Verification items for the finished model (mm, model axes). Face numbers are marked on the shaded views. A direction names the side the tool comes from. Coordinates: 2 decimals unless noted, no trailing zeros. Order: outer loops, then holes, each group sorted by start corner. A loop starts at its lowest first (then second) coordinate and runs counter-clockwise, first axis right, second up. Notation, with made-up numbers: M -28.5,81 L -10.5,81 A27 cw -10.5,97 Z; hole C -22,33 d7. An arc over 180 degrees is marked long. Return JSON: item names as keys, results as strings. Group by question number.
1. Material ranges on line 1 along Y through (x, z) = (10, 2.5); line 2 along X through (y, z) = (-5.5, 10.5); line 3 along X through (y, z) = (-2.5, 3.5), recorded low to high.
2. Section check C-C, the plane y = -2.25. Record the cut outline in (x, z), plus the area to 3 significant figures.
3. Mould release check, pull along Y, two halves, no side actions. Record for the marked faces 5, 6 and 7: +Y half, -Y half, draft (parallel to the pull), parting line (faces both ways), or undercut.
4. Section check D-D, the plane x = -2. Record the cut outline in (y, z).
5. Section check B-B, the plane z = 8. Record the cut outline in (x, y).
6. Section check A-A, the plane x = -9.5. Record the cut outline in (y, z).
7. Set-up check for the marked faces 1, 2, 3 and 4: record each of +Z, -Z, +X, -X, +Y, -Y from which the full face is reachable in a straight line by a thin tool's end or side.
8. Gauge pin test, flat ends, axial feed: pin 1 (3 mm diameter, centred on x = -3, y = 2, fed in from +Z); pin 2 (7 mm diameter, centred on y = -3, z = 11, fed in from -X); pin 3 (1.2 mm diameter, centred on x = -10.5, y = 5, fed in from +Z). Record the tip position at first contact, or that the pin passes through.
```python
from build123d import *

# Parameters (mm, degrees)
SKETCH1_W               = 23.3
SKETCH1_H               = 15.5
BOSS_EXTRUDE1_DEPTH     = 3
SKETCH2_W               = 15.5
SKETCH2_H               = 15.5
BOSS_EXTRUDE2_DEPTH     = 10.5
CUT_EXTRUDE1_DEPTH      = 8
CUT_EXTRUDE2_DEPTH      = 10
CUT_EXTRUDE2_DEPTH_BACK = 3
SKETCH4_R               = 1.5
SKETCH5_W               = 35.704226427
SKETCH5_H               = 23.298790068
CUT_EXTRUDE3_DEPTH      = 1.6


with BuildPart() as part:
    # Sketch1 → Boss-Extrude1 (new body)
    with BuildSketch(Plane.XY):
        Rectangle(SKETCH1_W, SKETCH1_H)
    extrude(amount=BOSS_EXTRUDE1_DEPTH)

    # Sketch2 → Boss-Extrude2 (add)
    with BuildSketch(Plane.XY.offset(3)):
        Rectangle(SKETCH2_W, SKETCH2_H)
    extrude(amount=BOSS_EXTRUDE2_DEPTH)

    # Sketch3 → Cut-Extrude1 (cut)
    with BuildSketch(Plane.XY.offset(13.5)):
        with BuildLine():
            Line((-2.5, 4.304165553), (-2.5, 5.178078794))
            ThreePointArc((-2.5, 5.178078794), (-4.065863992, 4.065863992), (-5.178078794, 2.5))
            Line((-5.178078794, 2.5), (-5.178078794, -2.5))
            ThreePointArc((-5.178078794, -2.5), (-4.065863992, -4.065863992), (-2.5, -5.178078794))
            Line((-2.5, -5.178078794), (-2.5, -3.82452247))
            Line((-2.5, -3.82452247), (2.5, -3.82452247))
            Line((2.5, -3.82452247), (2.5, -5.178078794))
            ThreePointArc((2.5, -5.178078794), (4.065863992, -4.065863992), (5.178078794, -2.5))
            Line((5.178078794, -2.5), (3.988610893, -2.5))
            Line((3.988610893, -2.5), (3.988610893, 2.5))
            Line((3.988610893, 2.5), (5.178078794, 2.5))
            ThreePointArc((5.178078794, 2.5), (4.065863992, 4.065863992), (2.5, 5.178078794))
            Line((2.5, 5.178078794), (2.5, 4.304165553))
            Line((2.5, 4.304165553), (-2.5, 4.304165553))
        make_face()
        with BuildLine():
            Line((-5.178078794, -2.5), (-5.178078794, 2.5))
            ThreePointArc((-5.178078794, 2.5), (-5.75, 0), (-5.178078794, -2.5))
        make_face()
        with BuildLine():
            ThreePointArc((-5.178078794, -2.5), (-5.75, 0), (-5.178078794, 2.5))
            Line((-5.178078794, 2.5), (-7.75, 2.5))
            Line((-7.75, 2.5), (-7.75, -2.5))
            Line((-7.75, -2.5), (-5.178078794, -2.5))
        make_face()
        with BuildLine():
            ThreePointArc((2.5, 5.178078794), (0, 5.75), (-2.5, 5.178078794))
            Line((-2.5, 5.178078794), (-2.5, 4.304165553))
            Line((-2.5, 4.304165553), (2.5, 4.304165553))
            Line((2.5, 4.304165553), (2.5, 5.178078794))
        make_face()
        with BuildLine():
            Line((2.5, 7.75), (-2.5, 7.75))
            Line((-2.5, 7.75), (-2.5, 5.178078794))
            ThreePointArc((-2.5, 5.178078794), (0, 5.75), (2.5, 5.178078794))
            Line((2.5, 5.178078794), (2.5, 7.75))
        make_face()
        with BuildLine():
            Line((7.75, 2.5), (5.178078794, 2.5))
            ThreePointArc((5.178078794, 2.5), (5.605196387, 1.28229227), (5.75, 0))
            ThreePointArc((5.75, 0), (5.605196387, -1.28229227), (5.178078794, -2.5))
            Line((5.178078794, -2.5), (7.75, -2.5))
            Line((7.75, -2.5), (7.75, 2.5))
        make_face()
        with BuildLine():
            ThreePointArc((5.75, 0), (5.605196387, 1.28229227), (5.178078794, 2.5))
            Line((5.178078794, 2.5), (3.988610893, 2.5))
            Line((3.988610893, 2.5), (3.988610893, -2.5))
            Line((3.988610893, -2.5), (5.178078794, -2.5))
            ThreePointArc((5.178078794, -2.5), (5.605196387, -1.28229227), (5.75, 0))
        make_face()
        with BuildLine():
            Line((-2.5, -3.82452247), (-2.5, -5.178078794))
            ThreePointArc((-2.5, -5.178078794), (0, -5.75), (2.5, -5.178078794))
            Line((2.5, -5.178078794), (2.5, -3.82452247))
            Line((2.5, -3.82452247), (-2.5, -3.82452247))
        make_face()
        with BuildLine():
            ThreePointArc((2.5, -5.178078794), (0, -5.75), (-2.5, -5.178078794))
            Line((-2.5, -5.178078794), (-2.5, -7.75))
            Line((-2.5, -7.75), (2.5, -7.75))
            Line((2.5, -7.75), (2.5, -5.178078794))
        make_face()
    extrude(amount=-CUT_EXTRUDE1_DEPTH, mode=Mode.SUBTRACT)

    # Sketch4 → Cut-Extrude2 (cut, two sides: drawn at the far end of the back side and taken through both)
    with BuildSketch(Plane.XY.offset(3).offset(-CUT_EXTRUDE2_DEPTH_BACK)):
        with Locations((0, 7.75)):
            Circle(SKETCH4_R)
        with Locations((7.75, 0)):
            Circle(SKETCH4_R)
        with BuildLine():
            Line((11.65, 1.5), (7.75, 1.5))
            ThreePointArc((7.75, 1.5), (8.810660172, 1.060660172), (9.25, 0))
            ThreePointArc((9.25, 0), (8.810660172, -1.060660172), (7.75, -1.5))
            Line((7.75, -1.5), (11.65, -1.5))
            Line((11.65, -1.5), (11.65, 1.5))
        make_face()
        with BuildLine():
            ThreePointArc((-7.75, -1.5), (-9.25, 0), (-7.75, 1.5))
            Line((-7.75, 1.5), (-11.65, 1.5))
            Line((-11.65, 1.5), (-11.65, -1.5))
            Line((-11.65, -1.5), (-7.75, -1.5))
        make_face()
        with BuildLine():
            Line((-7.75, -1.5), (-7.75, 1.5))
            ThreePointArc((-7.75, 1.5), (-9.25, 0), (-7.75, -1.5))
        make_face()
        with BuildLine():
            ThreePointArc((-6.25, 0), (-6.689339828, 1.060660172), (-7.75, 1.5))
            Line((-7.75, 1.5), (-7.75, -1.5))
            ThreePointArc((-7.75, -1.5), (-6.689339828, -1.060660172), (-6.25, 0))
        make_face()
        with Locations((0, -7.75)):
            Circle(SKETCH4_R)
    extrude(amount=CUT_EXTRUDE2_DEPTH + CUT_EXTRUDE2_DEPTH_BACK, mode=Mode.SUBTRACT)

    # Sketch5 → Cut-Extrude3 (cut)
    with BuildSketch(Plane(origin=(0, 0, 0), x_dir=(-1, 0, 0), z_dir=(0, 0, -1))):
        with Locations((1.840090656, -1.042081913)):
            Rectangle(SKETCH5_W, SKETCH5_H)
    extrude(amount=-CUT_EXTRUDE3_DEPTH, mode=Mode.SUBTRACT)


solid = part.part
```
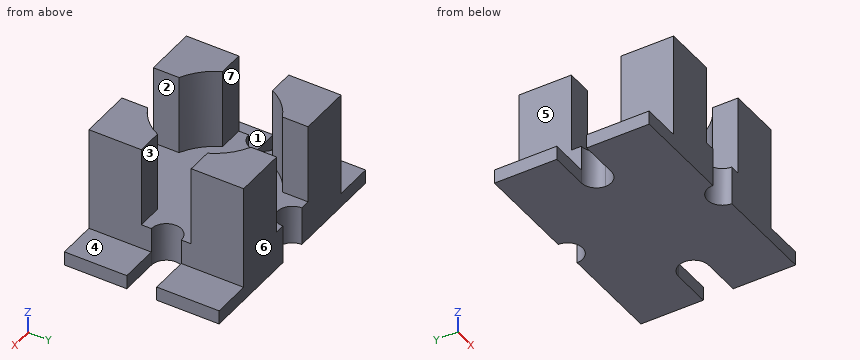
Answers follow:
{
 "1": {"line 1": "-7.75 to -1.5, 1.5 to 7.75", "line 2": "-7.75 to -2.5, 2.5 to 7.75", "line 3": "-7.75 to 7.75"},
 "2": {"outline": "M -11.65,1.6 L 11.65,1.6 L 11.65,3 L 7.75,3 L 7.75,5.5 L -7.75,5.5 L -7.75,3 L -11.65,3 Z", "area": "71.4 mm^2"},
 "3": {"face 5": "draft", "face 6": "+Y half", "face 7": "undercut"},
 "4": {"outline": "M -7.75,1.6 L 7.75,1.6 L 7.75,5.5 L -7.75,5.5 Z"},
 "5": {"outline": "M -7.75,-7.75 L -2.5,-7.75 L -2.5,-5.18 A5.75 cw -5.18,-2.5 L -7.75,-2.5 Z; M -7.75,2.5 L -5.18,2.5 A5.75 cw -2.5,5.18 L -2.5,7.75 L -7.75,7.75 Z; M 2.5,-7.75 L 7.75,-7.75 L 7.75,-2.5 L 5.18,-2.5 A5.75 cw 2.5,-5.18 Z; M 2.5,5.18 A5.75 cw 5.18,2.5 L 7.75,2.5 L 7.75,7.75 L 2.5,7.75 Z"},
 "6": {"outline": "M -7.75,1.6 L -1.5,1.6 L -1.5,3 L -7.75,3 Z; M 1.5,1.6 L 7.75,1.6 L 7.75,3 L 1.5,3 Z"},
 "7": {"face 1": "+Z, -X, +Y, -Y", "face 2": "+Z, +Y, -Y", "face 3": "+Z, +X, -X", "face 4": "+Z, +X, +Y, -Y"},
 "8": {"pin 1": "z = 5.5", "pin 2": "x = -7.75", "pin 3": "z = 3"}
}
